```python
from build123d import *

# Parameters (mm, degrees)
SKETCH1_W           = 33
SKETCH1_H           = 4
BOSS_EXTRUDE2_DEPTH = 300
CUT_EXTRUDE2_DEPTH  = 1
SKETCH5_R           = 2.25
CUT_EXTRUDE3_DEPTH  = 301.46838436
LPATTERN1_COUNT     = 10
LPATTERN1_PITCH     = 30


with BuildPart() as part:
    # Sketch1 → Boss-Extrude2 (new body)
    with BuildSketch(Plane.XY):
        Rectangle(SKETCH1_W, SKETCH1_H)
    extrude(amount=BOSS_EXTRUDE2_DEPTH)

    # Sketch2 → Cut-Extrude2 (cut)
    with BuildSketch(Plane(origin=(0, 2, 0), x_dir=(1, 0, 0), z_dir=(0, 1, 0))):
        with BuildLine():
            Line((-12.5, -10.875), (-16.5, -10.875))
            Line((-16.5, -10.875), (-16.5, -19.125))
            Line((-16.5, -19.125), (-12.5, -19.125))
            ThreePointArc((-12.5, -19.125), (-8.375, -15), (-12.5, -10.875))
        make_face()
    cut_extrude2 = extrude(amount=-CUT_EXTRUDE2_DEPTH, mode=Mode.SUBTRACT)

    # Sketch5 → Cut-Extrude3 (cut, through all)
    with BuildSketch(Plane(origin=(0, 1, 0), x_dir=(1, 0, 0), z_dir=(0, 1, 0))):
        with Locations(Location((-12.5, -15, 0), (0, 0, 270))):
            Circle(SKETCH5_R)
    cut_extrude3 = extrude(amount=-CUT_EXTRUDE3_DEPTH, mode=Mode.SUBTRACT)

    # LPattern1: Cut-Extrude2, Cut-Extrude3 ×10
    with Locations(*[(0, 0, i * LPATTERN1_PITCH) for i in range(1, LPATTERN1_COUNT)]):
        add(cut_extrude2, mode=Mode.SUBTRACT)
        add(cut_extrude3, mode=Mode.SUBTRACT)


solid = part.part
```
CAD build for the part. Positions are in the model's coordinates, mm. A direction names the side the tool comes from. Give positions to 0.01 mm unless a question says otherwise; leave off trailing zeros. Return JSON: item names as keys, results as strings. Group by question number.
(1) Drill centre lines: L1, parallel to X at y = 0.25, z = 285; L2, parallel to X at y = -1.15, z = 227; L3, parallel to X at y = 1.25, z = 77.5. Where is each one in solid material? Low to high. Write a range as [from, to].
(2) Mould opens along Z. For faces 1 (the face through (-14, 1, 17)), 2 (the face through (0, -2, 148)) say: pulls with the +Z half, pulls with the -Z half, needs draft (parallel to the pull), parting line crosses it, or undercut.
(3) Flat gauge pins, fed straight in: pin 1 Ø3.5 at (x, z) = (-12.5, 255) entering from +Y; pin 2 Ø2.5 at (x, z) = (-13.5, 167) entering from +Y. Where does each tip first touch, or does it go through?
(4) 3-axis set-ups, long thin cutter, end or side, ignore diameter. For faces 3 (the face through (-14, 1, 167)), 4 (the face through (0, 2, 148)): which of +Z, -Z, +X, -X, +Y, -Y reach the whole face in a straight line?
(5) Band-saw the part on A-A (y = 0.15). State how many separate pieces and enclosed holes the cut face has, and give its area (3 significant figures).
Entries:
{
 "1": {"L1": "x = [-16.5, -14.75], [-10.25, 16.5]", "L2": "x = [-16.5, -13.53], [-11.47, 16.5]", "L3": "x = [-9.22, 16.5]"},
 "2": {"face 1": "undercut", "face 2": "needs draft"},
 "3": {"pin 1": "passes through", "pin 2": "stops at y = 1"},
 "4": {"face 3": "-X, +Y", "face 4": "+Z, -Z, +X, -X, +Y"},
 "5": {"separate pieces": "1", "enclosed holes": "10", "area": "9,740 mm^2"}
}
